Autodesk Inventor part; units mm, degrees
ref_plane "Work Plane1" through (15, 0, 0) normal (1, 0, 0) x (0, 1, 0)
ref_plane "YZ Plane" through (0, 0, 0) normal (1, 0, 0) x (0, 1, 0)
ref_plane "XZ Plane" through (0, 0, 0) normal (0, 1, 0) x (-1, 0, 0)
sketch "Sketch1" plane through (0, 0, 0) normal (0, 0, 1) x (1, 0, 0)
  line L0 (0, 0) -> (0, 6)
  line L1 (0, 6) -> (15, 6)
  line L2 (15, 6) -> (15, 6)
  line L3 (15, 6) -> (40, 6)
  line L4 (40, 6) -> (40, 6)
  line L5 (40, 6) -> (70, 6)
  line L6 (70, 6) -> (70, 0)
  line L7 (70, 0) -> (0, 0)
  dimension "d1" = 12
  dimension "d3" = 12
  dimension "d4" = 15
  dimension "d5" = 55
  dimension "d6" = 30
revolve "Revolution1" add sketch "Sketch1" angle 360 about axis through (70, 0, 0) along (-1, 0, 0)
thread "Thread1"
thread "Thread2"
chamfer "Chamfer1" distance 0.8 angle 45 2 edges at (70, -6, 0) (0, -6, 0)
ref_plane "Work Plane1" through (15, 0, 0) normal (1, 0, 0) x (0, 1, 0)
sketch "Sketch2" plane through (15, 0, 0) normal (1, 0, 0) x (0, 1, 0)
  circle A0 centre (0, 0) radius 6
  point P0 (0, 0)
  dimension "d29" = 12
boundary_patch "Boundary Patch1"
equation "\"d8\" = d4"
equation "\"d23\" = b"
equation "\"d25\" = chamfer"
equation "\"d1\" = d"
equation "\"d3\" = d1_"
equation "\"d4\" = b1"
equation "\"d5\" = L"
equation "\"d6\" = b"
equation "\"d29\" = d"
equation "\"chamfer\" = 0.8"
equation "\"d\" = 12"
equation "\"d1_\" = 12"
equation "\"b1\" = 15"
equation "\"L\" = 55"
equation "\"b\" = 30"
equation "\"d28\" = -b1"
equation "\"Grip_Length\" = 25"
properties part number "Stud M12-6g×55 GOST 22034-76" material "Steel, Mild"
Geometry check sheet. Reference: the model listing, model coordinates, mm. Give positions to 0.01 mm unless a question says otherwise; leave off trailing zeros. Order: outer loops, then holes, each group sorted by start corner. A loop starts at its lowest first (then second) coordinate and runs counter-clockwise, first axis right, second up. Notation, with made-up numbers: (25, -39) - (69, -39) arc R35 cw to (69, 0) - close; hole circle Ø2 at (35, 13). An arc over 180 degrees is marked (long way). Use one line per item in the form item = value.
1) Depth check by flat-ended pin: pin 1 Ø3 at (x, y) = (59, -3.5) entering from -Z. Enter the tip coordinate at first touch or a pass-through.
Working result:
pin_1 = -5.66
2) Material ranges on probe 1 along Y at (x, z) = (25.5, -3); probe 2 along Y at (x, z) = (36, 2.75), recorded low to high. Write a range as from..to.
Working result:
probe_1 = -5.2..5.2
probe_2 = -5.33..5.33
3) Sectioned sample at A-A (x = 47). Record the boundary of the cut face in (y, z).
Working result:
outline = circle Ø12 at (0, 0)
